Read the model definition and answer for the solid it produces. Units are mm, in the model's axes. Coordinates: 2 decimals unless noted, no trailing zeros. Loops run counter-clockwise (first coordinate to the right, second up) from the corner with the lowest first, then second, coordinate; pieces in that order, holes last. Notation, with made-up numbers: (56.25, -38) -> (91.25, -38) arc R30 cw to (91.25, -14) -> close; hole circle Ø3 at (17.25, -19.5). An arc over 180 degrees is marked (long way). Answer as a JSON object with one key per item and string values. Group by question number.
1) Consider probe 1 along X at (y, z) = (0.75, 659.13); probe 2 along X at (y, z) = (15, 638.5). Determine where each line is inside the solid, lowest interval first. Write a range as [from, to].
2) Section A-A, the plane y = 14.25 is taken. Give the vertices of the cut face in (x, z).
3) Flat-ended cylindrical pins translate along their axes: P1, Ø12, axis at y = 4.5, z = 348, coming from the -X side; P2, Ø8, axis at x = 10.5, y = 3.5, coming from the +Z side. Find the tip coordinate at first contact, or state that the pin passes through.
4) Section B-B, the plane z = 190.5 is taken. Give the vertices of the cut face in (x, y).
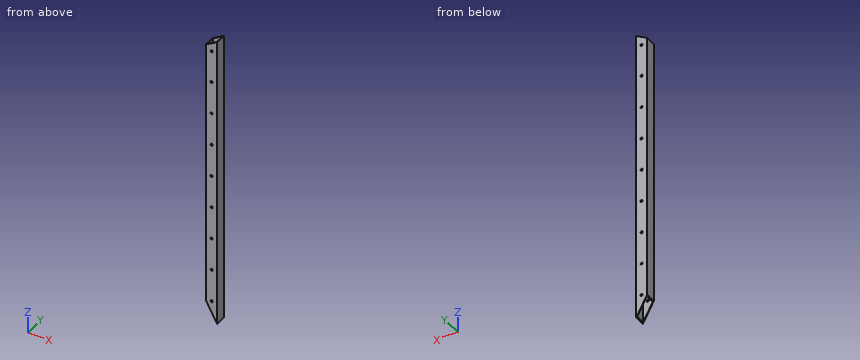
from build123d import *

# Parameters (mm, degrees)
SKETCH1_W           = 25.4
SKETCH1_H           = 25.4
SKETCH1_W_2         = 22.225
SKETCH1_H_2         = 22.225
BOSS_EXTRUDE1_DEPTH = 685.8
SKETCH3_R           = 2.54
CUT_EXTRUDE2_DEPTH  = 687.740096397


with BuildPart() as part:
    # Sketch1 → Boss-Extrude1 (new body)
    with BuildSketch(Plane.XY):
        with Locations((12.7, 12.7)):
            Rectangle(SKETCH1_W, SKETCH1_H)
        with Locations((12.7, 12.7)):
            Rectangle(SKETCH1_W_2, SKETCH1_H_2, mode=Mode.SUBTRACT)
    extrude(amount=BOSS_EXTRUDE1_DEPTH)

    # Sketch3 → Cut-Extrude2 (cut, through all)
    with BuildSketch(Plane(origin=(0, 25.4, 0), x_dir=(1, 0, 0), z_dir=(0, 1, 0))):
        with Locations(Location((12.7, -50.8, 0), (0, 0, 270))):
            Circle(SKETCH3_R)
        with Locations(Location((12.7, -127, 0), (0, 0, 270))):
            Circle(SKETCH3_R)
        with Locations(Location((12.7, -203.2, 0), (0, 0, 270))):
            Circle(SKETCH3_R)
        with Locations(Location((12.7, -279.4, 0), (0, 0, 270))):
            Circle(SKETCH3_R)
        with Locations(Location((12.7, -355.6, 0), (0, 0, 270))):
            Circle(SKETCH3_R)
        with Locations(Location((12.7, -431.8, 0), (0, 0, 270))):
            Circle(SKETCH3_R)
        with Locations(Location((12.7, -508, 0), (0, 0, 270))):
            Circle(SKETCH3_R)
        with Locations(Location((12.7, -584.2, 0), (0, 0, 270))):
            Circle(SKETCH3_R)
        with Locations(Location((12.7, -659.13, 0), (0, 0, 270))):
            Circle(SKETCH3_R)
        Polygon((0, 0), (0, -46.780980505), (25.4, 0), align=None)
        Polygon((0, -685.8), (0, -671.720550093), (25.4, -685.8), align=None)
    extrude(amount=-CUT_EXTRUDE2_DEPTH, mode=Mode.SUBTRACT)


solid = part.part
Determined:
{
 "1": {"probe 1": "[0, 10.16], [15.24, 25.4]", "probe 2": "[0, 1.59], [23.81, 25.4]"},
 "2": {"outline": "(0, 46.78) -> (1.59, 43.86) -> (1.59, 672.6) -> (0, 671.72) -> close; (23.81, 2.92) -> (25.4, 0) -> (25.4, 685.8) -> (23.81, 684.92) -> close"},
 "3": {"P1": "x = 0", "P2": "z = 679.49"},
 "4": {"outline": "(0, 0) -> (25.4, 0) -> (25.4, 25.4) -> (0, 25.4) -> close; hole (1.59, 1.59) -> (23.81, 1.59) -> (23.81, 23.81) -> (1.59, 23.81) -> close"}
}
